Input: part model. Units: mm. Frame: model coordinates. A direction names the side the tool comes from. Coordinates: 2 decimals unless noted, no trailing zeros. Order: outer loops, then holes, each group sorted by start corner. A loop starts at its lowest first (then second) coordinate and runs counter-clockwise, first axis right, second up. Notation, with made-up numbers: (29.5, 89.5) - (61.5, 89.5) arc R9 cw to (61.5, 98.5) - close; hole circle Ø9 at (74.25, 82). An arc over 180 degrees is marked (long way). Use a Markdown table: item, result. Add a question column.
from build123d import *
from build123d.topology import SkipClean

# Parameters (mm, degrees)
BASPROSKE_W         = 8
BASPROSKE_H         = 5.75
TOOTHCUT_DEPTH      = 12.407234547
TEETHCUTS_COUNT     = 21
TEETHCUTS_ANGLE     = 342.857142857
HUBNEARONE_START    = 8.0000508
HUBNEAONESKE_R      = 4.624
HUBNEARONE_DEPTH    = 8.0000508
BORSKE_R            = 2.5
BORE_DEPTH          = 16.0000508
SKETCH1_R           = 9
SKETCH1_R_2         = 4.624
BOSS_EXTRUDE1_DEPTH = 8.0000508
SKETCH3_R           = 1.8
CUT_EXTRUDE1_DEPTH  = 16.033323412
SKETCH4_W           = 5.5
SKETCH4_H           = 2.2
CUT_EXTRUDE2_DEPTH  = 5.5


with BuildPart() as part:
    # BasProSke → Base-Revolve (revolve)
    with BuildSketch(Plane(origin=(0, 0, 0), x_dir=(1, 0, 0), z_dir=(0, 1, 0)), mode=Mode.PRIVATE) as base_revolve_sk:
        with Locations((4, 2.875)):
            Rectangle(BASPROSKE_W, BASPROSKE_H)
    revolve(base_revolve_sk.sketch.rotate(Axis((-10, 0, 0), (1, 0, 0)), 180), axis=Axis((-10, 0, 0), (1, 0, 0)))

    # TooCutSke → ToothCut (cut, through all)
    with BuildSketch(Plane(origin=(0, 0, 0), x_dir=(0, 0, -1), z_dir=(1, 0, 0))):
        with BuildLine():
            ThreePointArc((0.247570178, 4.617367757), (0, 4.624), (-0.247570178, 4.617367757))
            ThreePointArc((-0.247570178, 4.617367757), (-0.414765128, 5.209076442), (-0.746177874, 5.726994302))
            ThreePointArc((-0.746177874, 5.726994302), (0, 5.7754), (0.746177874, 5.726994302))
            ThreePointArc((0.746177874, 5.726994302), (0.414765128, 5.209076442), (0.247570178, 4.617367757))
        make_face()
    toothcut = extrude(amount=TOOTHCUT_DEPTH, mode=Mode.SUBTRACT)

    # TeethCuts: ToothCut ×21 about axis
    teethcuts_axis = Axis((-10, 0, 0), (1, 0, 0))
    for i in range(1, TEETHCUTS_COUNT):
        add(toothcut.rotate(teethcuts_axis, i * TEETHCUTS_ANGLE / (TEETHCUTS_COUNT - 1)), mode=Mode.SUBTRACT)

    # HubNeaOneSke → HubNearOne (add)
    with SkipClean():  # the faces are left unmerged after this step: merging them gives an invalid solid
        with BuildSketch(Plane.ZY.offset(HUBNEARONE_START)):
            Circle(HUBNEAONESKE_R)
        extrude(amount=-HUBNEARONE_DEPTH)

    # BorSke → Bore (cut, symmetric)
    with SkipClean():  # the faces are left unmerged after this step: merging them gives an invalid solid
        with BuildSketch(Plane(origin=(0, 0, 0), x_dir=(0, 0, -1), z_dir=(1, 0, 0))):
            with Locations(Location((0, 0, 0), (0, 0, 180))):
                Circle(BORSKE_R)
        extrude(amount=BORE_DEPTH, both=True, mode=Mode.SUBTRACT)

    # Sketch1 → Boss-Extrude1 (add)
    with BuildSketch(Plane.ZY.offset(8.0000508)):
        Circle(SKETCH1_R)
        Circle(SKETCH1_R_2, mode=Mode.SUBTRACT)
    extrude(amount=-BOSS_EXTRUDE1_DEPTH)

    # Sketch3 → Cut-Extrude1 (cut, through all)
    with BuildSketch(Plane(origin=(0, 0, 0), x_dir=(1, 0, 0), z_dir=(0, 1, 0))):
        with Locations(Location((-5.2500508, 0, 0), (0, 0, 270))):
            Circle(SKETCH3_R)
    extrude(amount=-CUT_EXTRUDE1_DEPTH, mode=Mode.SUBTRACT)

    # Sketch4 → Cut-Extrude2 (cut)
    with BuildSketch(Plane.ZY.offset(8.0000508)):
        with Locations((0, -5)):
            Rectangle(SKETCH4_W, SKETCH4_H)
    extrude(amount=-CUT_EXTRUDE2_DEPTH, mode=Mode.SUBTRACT)


solid = part.part
1) Cut plane B-B (z = 7.5). Return the cut outline in (x, y).
2) Contact query for flat-ended pins moving along their axis: P1, Ø5, axis at x = 5.5, z = 1, coming from the +Y side; P2, Ø1.8, axis at y = -5, z = 0, coming from the -X side; P3, Ø0.7, axis at x = -5, y = -5.5, coming from the +Z side; P4, Ø4.5, axis at y = 0, z = 0, coming from the +X side. Output: stop coordinate, or through.
3) Cut plane A-A (y = 2.25). Return the cut outline in (x, z), and give its area (3 significant figures).
4) Material intervals for L1, parallel to Z at x = 0.25, y = -4.75; L2, parallel to Z at x = 6.75, y = -3.5; L3, parallel to Y at x = 3.5, z = 5.25, sorted ascending.
5) Pull-direction query (Z, two-part tool) for faces 1 (the flat face through (-8, 2, 2)), 2 (the flat face through (-2.5, -5, 0)); classes: pulls with the +Z half, pulls with the -Z half, needs draft (parallel to the pull), parting line crosses it, or undercut.
6) Reachability of faces 3 (the cylindrical face through (0.11, 2.44, -0.54)), 4 (the cylindrical face through (3.94, 2.92, -4.32)), 5 (the cylindrical face through (3.944, 5.187, 0.405)), 6 (the cylindrical face through (3.94, -4.51, 2.63)), 7 (the flat face through (-5, -5, 2.75)) from +Z, -Z, +X, -X, +Y, -Y: full face, straight path, thin tool, end or side. Return the list, or none.
Computed:
| question | item | result |
|---|---|---|
| 1 | outline | (-8, -4.97) - (0, -4.97) - (0, 4.97) - (-8, 4.97) - close |
| 2 | P1 | stops at y = 5.7 |
| 2 | P2 | stops at x = -2.5 |
| 2 | P3 | stops at z = 7.38 |
| 2 | P4 | passes through |
| 3 | outline | (-8, -8.71) - (0, -8.71) - (0, -4.66) - (8, -4.66) - (8, -1.09) - (-8, -1.09) - close; (-8, 1.09) - (8, 1.09) - (8, 4.66) - (0, 4.66) - (0, 8.71) - (-8, 8.71) - close |
| 3 | area | 179 mm2 |
| 4 | L1 | z = -3.24 to -2.98, -1.88 to -1.01, -0.44 to 0.44, 1.01 to 1.88, 2.98 to 3.24 |
| 4 | L2 | z = -4.56 to -3.77, -3.02 to 3.02, 3.77 to 4.56 |
| 4 | L3 | y = -2.23 to -1.8, -0.74 to -0.03, 0.85 to 1.49 |
| 5 | face 1 | needs draft |
| 5 | face 2 | undercut |
| 6 | face 3 | +X, -X |
| 6 | face 4 | +X |
| 6 | face 5 | +X, +Y |
| 6 | face 6 | +X, -Y |
| 6 | face 7 | -X |
